Design review of the part built by this model. Coordinates are the model's own, in mm. Give positions to 0.01 mm unless a question says otherwise; leave off trailing zeros. Write each loop counter-clockwise with the first axis right and the second up, starting at its lowest first coordinate (ties: lowest second). Pieces come first, ordered by that corner, then holes. Notation, with made-up numbers: (41.25, 1.5) -> (94.25, 1.5) arc R19 ccw to (94.25, 10.5) -> close; hole circle Ø9 at (76.5, 60.5). An arc over 180 degrees is marked (long way). Put each result on its own line as item: value. Start each with the question number.
from build123d import *

# Parameters (mm, degrees)
SKETCH1_R           = 7.5
BOSS_EXTRUDE1_DEPTH = 36.206884
SKETCH2_R           = 4.299113173
CUT_EXTRUDE1_DEPTH  = 38.728483259
CHAMFER1_SIZE       = 1.210647


with BuildPart() as part:
    # Sketch1 → Boss-Extrude1 (new body)
    with BuildSketch(Plane(origin=(0, 0, 0), x_dir=(1, 0, 0), z_dir=(0, 1, 0))):
        with Locations(Location((0, 0, 0), (0, 0, 270))):
            Circle(SKETCH1_R)
    extrude(amount=BOSS_EXTRUDE1_DEPTH)

    # Sketch2 → Cut-Extrude1 (cut, through all)
    with BuildSketch(Plane(origin=(0, 0, 0), x_dir=(1, 0, 0), z_dir=(0, 1, 0))):
        with Locations(Location((0, 0, 0), (0, 0, 270))):
            Circle(SKETCH2_R)
    extrude(amount=CUT_EXTRUDE1_DEPTH, mode=Mode.SUBTRACT)

    # Chamfer1
    chamfer1_edges = [part.edges().sort_by_distance(p)[0] for p in [
        (0, 0, -7.5),
        (0, 36.206884, -7.5),
        (0, 0, -4.299113173),
        (0, 36.206884, -4.299113173),
    ]]
    chamfer(chamfer1_edges, length=CHAMFER1_SIZE)


solid = part.part
Q1. For pin 1 (5 mm diameter, centred on x = -4, z = 6, fed in from -Y); pin 2 (6 mm diameter, centred on x = 4, y = 27.5, fed in from +Z); pin 3 (2 mm diameter, centred on x = -2.5, y = 15, fed in from +Z); pin 4 (1 mm diameter, centred on x = -0.5, z = 3.5, fed in from -Y), all flat-tipped, find the tip position at first contact; note any pin that passes through.
Q2. Take a section at C-C on y = 26. Give the boundary of the cut face in (x, z).
Q3. Mouldability with a two-part tool opening along Z and no side actions: class faces 1 (the face through (0.33, 17.867, -7.493)), 2 (the face through (-6, 36.207, 0)), 3 (the face through (4.263, 17.867, -0.56)) as +Z half, -Z half, draft (parallel to the pull), parting line (faces both ways), or undercut.
Q4. Take a section at B-B on x = 0. Give the boundary of the cut face in (y, z), then the cut area to 3 significant figures.
Q5. Take a section at A-A on z = 0. Give the boundary of the cut face in (x, y), then the cut area to 3 significant figures.
Q6. To check wall thickness, follow probe 1 along X at (y, z) = (10.5, 0); probe 2 along Z at (x, y) = (-0.25, 2); probe 3 along X at (y, z) = (9, 3.5). State the ranges of each line that lie inside material, in increasing order. Write a range as from..to.
Result:
1. pin 1: stops at y = 0
1. pin 2: stops at z = 7.43
1. pin 3: stops at z = 7.35
1. pin 4: passes through
2. outline: circle Ø15 at (0, 0); hole circle Ø8.6 at (0, 0)
3. face 1: parting line
3. face 2: draft
3. face 3: undercut
4. outline: (0, -6.29) -> (1.21, -7.5) -> (35, -7.5) -> (36.21, -6.29) -> (36.21, -5.51) -> (35, -4.3) -> (1.21, -4.3) -> (0, -5.51) -> close; (0, 5.51) -> (1.21, 4.3) -> (35, 4.3) -> (36.21, 5.51) -> (36.21, 6.29) -> (35, 7.5) -> (1.21, 7.5) -> (0, 6.29) -> close
4. area: 226 mm^2
5. outline: (-7.5, 1.21) -> (-6.29, 0) -> (-5.51, 0) -> (-4.3, 1.21) -> (-4.3, 35) -> (-5.51, 36.21) -> (-6.29, 36.21) -> (-7.5, 35) -> close; (4.3, 1.21) -> (5.51, 0) -> (6.29, 0) -> (7.5, 1.21) -> (7.5, 35) -> (6.29, 36.21) -> (5.51, 36.21) -> (4.3, 35) -> close
5. area: 226 mm^2
6. probe 1: x = -7.5..-4.3, 4.3..7.5
6. probe 2: z = -7.5..-4.29, 4.29..7.5
6. probe 3: x = -6.63..-2.5, 2.5..6.63
